Design review of the part built by this model. Coordinates are the model's own, in mm. Coordinates: 2 decimals unless noted, no trailing zeros. Write each loop counter-clockwise with the first axis right and the second up, starting at its lowest first coordinate (ties: lowest second). Pieces come first, ordered by that corner, then holes. Notation, with made-up numbers: (23.25, -38.5) -> (71.25, -38.5) arc R25 ccw to (71.25, -7.5) -> close; hole circle Ø9 at (-26.5, -17). An arc over 180 degrees is marked (long way). Write item = value, one per line. Start each with the question number.
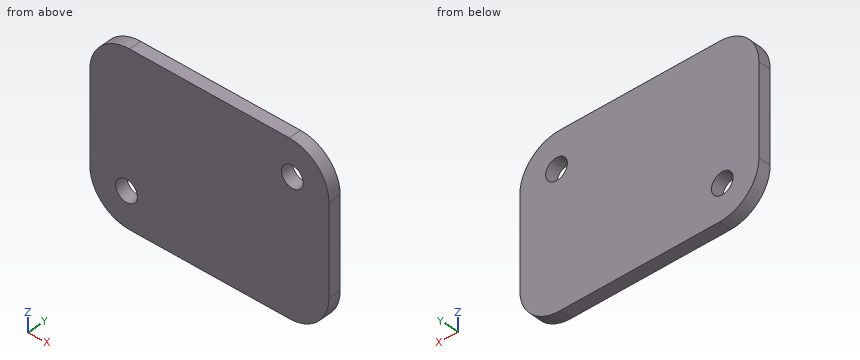
```python
from build123d import *

# Parameters (mm, degrees)
BOSS_EXTRUDE1_DEPTH             = 3.175
F_7_32_0_21875_DIAMETER_HOLE1_D = 5.55625


with BuildPart() as part:
    # Sketch1 → Boss-Extrude1 (new body)
    with BuildSketch(Plane(origin=(0, 0, 0), x_dir=(1, 0, 0), z_dir=(0, 1, 0))):
        with BuildLine():
            Line((-20.447, -21.717), (20.447, -21.717))
            ThreePointArc((20.447, -21.717), (27.631204897, -18.741204897), (30.607, -11.557))
            Line((30.607, -11.557), (30.607, 11.557))
            ThreePointArc((30.607, 11.557), (27.631204897, 18.741204897), (20.447, 21.717))
            Line((20.447, 21.717), (-20.447, 21.717))
            ThreePointArc((-20.447, 21.717), (-27.631204897, 18.741204897), (-30.607, 11.557))
            Line((-30.607, 11.557), (-30.607, -11.557))
            ThreePointArc((-30.607, -11.557), (-27.631204897, -18.741204897), (-20.447, -21.717))
        make_face()
    extrude(amount=BOSS_EXTRUDE1_DEPTH)

    # 7/32 (0.21875) Diameter Hole1 (through all)
    with Locations(Plane(origin=(0, 3.175, 0), x_dir=(1, 0, 0), z_dir=(0, 1, 0))):
        with Locations((-21.214511478, 12.776921686), (21.214511478, -12.776921686)):
            Hole(F_7_32_0_21875_DIAMETER_HOLE1_D / 2)


solid = part.part
```
(1) Take a section at A-A, the plane z = 14.5. State the section outline as (x, y) points (3 decimals), then the cut area to 3 significant figures.
(2) For pin 1 Ø1 at (x, y) = (24, 1.5) entering from +Z, flat-tipped, find the tip position at first contact; note if it passes through.
(3) Take a section at B-B, the plane x = -19.5. State the section outline as (y, z) points (3 decimals), then the cut area to 3 significant figures.
(4) Take a section at C-C, the plane y = 2.6. State the section outline as (x, z) points, then the cut area to 3 significant figures.
(5) Take a section at D-D, the plane z = -19. State the section outline as (x, y) points (3 decimals), then the cut area to 3 significant figures.
(6) For line 1 (X direction, y = 1.9, z = -12.5); line 2 (Z direction, x = -23, y = 1.8); line 3 (X direction, y = 0.45, z = -15), list the stretches that pass through material, from the lowest coordinate up.
Report:
q1.outline = (-30.171, 0) -> (19.035, 0) -> (19.035, 3.175) -> (-30.171, 3.175) -> close; (23.394, 0) -> (30.171, 0) -> (30.171, 3.175) -> (23.394, 3.175) -> close
q1.area = 178 mm2
q2.pin_1 = 21.25
q3.outline = (0, -21.717) -> (3.175, -21.717) -> (3.175, -14.963) -> (0, -14.963) -> close; (0, -10.591) -> (3.175, -10.591) -> (3.175, 21.717) -> (0, 21.717) -> close
q3.area = 124 mm2
q4.outline = (-30.61, -11.56) arc R10.16 ccw to (-20.45, -21.72) -> (20.45, -21.72) arc R10.16 ccw to (30.61, -11.56) -> (30.61, 11.56) arc R10.16 ccw to (20.45, 21.72) -> (-20.45, 21.72) arc R10.16 ccw to (-30.61, 11.56) -> close; hole circle Ø5.56 at (-21.21, -12.78); hole circle Ø5.56 at (21.21, 12.78)
q4.area = 2,520 mm2
q5.outline = (-27.363, 0) -> (27.363, 0) -> (27.363, 3.175) -> (-27.363, 3.175) -> close
q5.area = 174 mm2
q6.line_1 = -30.56 to -23.98, -18.45 to 30.56
q6.line_2 = -21.39 to -14.91, -10.65 to 21.39
q6.line_3 = -30.01 to -22.88, -19.55 to 30.01
